For this review, take the finished solid that the model builds, in its own axes (mm). A direction names the side the tool comes from. Round coordinates to 2 decimals unless told otherwise and drop trailing zeros. Loops run counter-clockwise (first coordinate to the right, second up) from the corner with the lowest first, then second, coordinate; pieces in that order, holes last. Notation, with made-up numbers: (40.5, -34) -> (75.5, -34) arc R18 cw to (75.5, -22) -> close; hole circle Ø1 at (50, 12). An arc over 180 degrees is marked (long way). Write each question's results on one line, items separated by ' | '.
```python
from build123d import *

# Parameters (mm, degrees)
SKETCH2_W           = 406.4
SKETCH2_H           = 101.6
BOSS_EXTRUDE2_DEPTH = 2.54
SKETCH3_R           = 4.826
CUT_EXTRUDE1_DEPTH  = 2.54
SKETCH4_R           = 3.937
CUT_EXTRUDE2_DEPTH  = 2.54
SKETCH5_W           = 12.7
SKETCH5_H           = 76.2
BOSS_EXTRUDE4_DEPTH = 12.7


with BuildPart() as part:
    # Sketch2 → Boss-Extrude2 (new body)
    with BuildSketch(Plane.XY):
        Rectangle(SKETCH2_W, SKETCH2_H)
    extrude(amount=-BOSS_EXTRUDE2_DEPTH)

    # Sketch3 → Cut-Extrude1 (cut)
    with BuildSketch(Plane.XY):
        with Locations((-44.45, 44.45)):
            Circle(SKETCH3_R)
        with Locations((44.45, 44.45)):
            Circle(SKETCH3_R)
        with Locations((44.45, -44.45)):
            Circle(SKETCH3_R)
        with Locations((-44.45, -44.45)):
            Circle(SKETCH3_R)
    extrude(amount=-CUT_EXTRUDE1_DEPTH, mode=Mode.SUBTRACT)

    # Sketch4 → Cut-Extrude2 (cut)
    with BuildSketch(Plane.XY):
        Circle(SKETCH4_R)
    extrude(amount=-CUT_EXTRUDE2_DEPTH, mode=Mode.SUBTRACT)

    # Sketch5 → Boss-Extrude4 (add)
    with BuildSketch(Plane.XY):
        with Locations((-184.15, 0)):
            Rectangle(SKETCH5_W, SKETCH5_H)
    boss_extrude4 = extrude(amount=-BOSS_EXTRUDE4_DEPTH)

    # Mirror2: Boss-Extrude4 across plane
    add(boss_extrude4.mirror(Plane(origin=(0, 0, 0), x_dir=(0, 0, 1), z_dir=(1, 0, 0))))


solid = part.part
```
1. To check wall thickness, follow probe 1 along Y at (x, z) = (-44.45, -1.1); probe 2 along X at (y, z) = (22, -7); probe 3 along X at (y, z) = (-42.5, -1.75). State the ranges of each line that lie inside material, in increasing order.
Values found:
probe 1: y = -50.8 to -49.28, -39.62 to 39.62, 49.28 to 50.8 | probe 2: x = -190.5 to -177.8, 177.8 to 190.5 | probe 3: x = -203.2 to -48.86, -40.04 to 40.04, 48.86 to 203.2
2. Tool access review of faces 1 (the face through (184, -38.1, -8)), 2 (the face through (177.8, -1, -8)), 3 (the face through (184, 38.1, -8)): name each direction out of +Z, -Z, +X, -X, +Y, -Y from which nothing blocks a thin tool from reaching the whole face with its end or side.
Values found:
face 1: -Z, +X, -X, -Y | face 2: -Z, +Y, -Y | face 3: -Z, +X, -X, +Y
3. Consider section A-A (y = 44.45). State the section outline as (x, z) points, plus the area to 3 significant figures.
Values found:
outline: (-203.2, -2.54) -> (-49.28, -2.54) -> (-49.28, 0) -> (-203.2, 0) -> close; (-39.62, -2.54) -> (39.62, -2.54) -> (39.62, 0) -> (-39.62, 0) -> close; (49.28, -2.54) -> (203.2, -2.54) -> (203.2, 0) -> (49.28, 0) -> close | area: 983 mm2
4. Draft analysis for pull direction X (two halves, no side actions). For faces 4 (the face through (3, -11, 0)), 5 (the face through (-0.853, -3.843, -1.252)), 6 (the face through (-190.5, -1, -8)), state which applies: released by +X, released by -X, zero draft, split by the parting line, or undercut.
Values found:
face 4: zero draft | face 5: undercut | face 6: released by -X
5. Consider section C-C (z = -8.25). State the section outline as (x, y) points, plus the area to 3 significant figures.
Values found:
outline: (-190.5, -38.1) -> (-177.8, -38.1) -> (-177.8, 38.1) -> (-190.5, 38.1) -> close; (177.8, -38.1) -> (190.5, -38.1) -> (190.5, 38.1) -> (177.8, 38.1) -> close | area: 1,940 mm2
6. Consider section B-B (x = 0). State the section outline as (y, z) points, plus the area to 3 significant figures.
Values found:
outline: (-50.8, -2.54) -> (-3.94, -2.54) -> (-3.94, 0) -> (-50.8, 0) -> close; (3.94, -2.54) -> (50.8, -2.54) -> (50.8, 0) -> (3.94, 0) -> close | area: 238 mm2
7. Consider section D-D (x = 44.45). State the section outline as (y, z) points, plus the area to 3 significant figures.
Values found:
outline: (-50.8, -2.54) -> (-49.28, -2.54) -> (-49.28, 0) -> (-50.8, 0) -> close; (-39.62, -2.54) -> (39.62, -2.54) -> (39.62, 0) -> (-39.62, 0) -> close; (49.28, -2.54) -> (50.8, -2.54) -> (50.8, 0) -> (49.28, 0) -> close | area: 209 mm2
8. For pin 1 (5 mm diameter, centred on y = -18.5, z = -9.5, fed in from -X); pin 2 (3 mm diameter, centred on x = -184, z = -10, fed in from +Y); pin 3 (15.5 mm diameter, centred on x = -44.45, y = 44.45, fed in from -Z), all flat-tipped, find the tip position at first contact; note any pin that passes through.
Values found:
pin 1: stops at x = -190.5 | pin 2: stops at y = 38.1 | pin 3: stops at z = -2.54
